```python
from build123d import *

# Parameters (mm, degrees)
SKETCH2_R           = 4.7625
BOSS_EXTRUDE1_DEPTH = 203.2
BOSS_EXTRUDE2_REACH = 30.575
SKETCH1_R           = 4.7625


with BuildPart() as part:
    # Sketch2 → Boss-Extrude1 (new body, symmetric)
    with BuildSketch(Plane(origin=(0, 0, 0), x_dir=(0, 0, -1), z_dir=(1, 0, 0))):
        with Locations((-23.8125, 0)):
            Circle(SKETCH2_R)
    extrude(amount=BOSS_EXTRUDE1_DEPTH, both=True)

    # Sketch1 → Boss-Extrude2 (add, up to next)
    with BuildSketch(Plane.XY, mode=Mode.PRIVATE) as boss_extrude2_sk1:
        with Locations((-155.575, 0)):
            Circle(SKETCH1_R)
    boss_extrude2_tool1 = extrude(boss_extrude2_sk1.sketch, amount=BOSS_EXTRUDE2_REACH, mode=Mode.PRIVATE) - part.part
    add(boss_extrude2_tool1.solids().sort_by_distance((-155.575, 0, 0))[0])
    # Sketch1 → Boss-Extrude2 (add, up to next)
    with BuildSketch(Plane.XY, mode=Mode.PRIVATE) as boss_extrude2_sk2:
        with Locations((155.575, 0)):
            Circle(SKETCH1_R)
    boss_extrude2_tool2 = extrude(boss_extrude2_sk2.sketch, amount=BOSS_EXTRUDE2_REACH, mode=Mode.PRIVATE) - part.part
    add(boss_extrude2_tool2.solids().sort_by_distance((155.575, 0, 0))[0])


solid = part.part
```
Work out the finished part from the listing and answer in its coordinate system (mm). A direction names the side the tool comes from. Coordinates: 2 decimals unless noted, no trailing zeros. Loops run counter-clockwise (first coordinate to the right, second up) from the corner with the lowest first, then second, coordinate; pieces in that order, holes last. Notation, with made-up numbers: (-18, 55) -> (-8, 55) arc R26 ccw to (-8, 84) -> close; hole circle Ø10 at (22.5, 65). An arc over 180 degrees is marked (long way). Answer as CSV lines item,"result".
Q1. A tool of negligible diameter and unlimited length cuts with its end or side. For faces 4 (the face through (2.84, 0.21, 28.57)), 5 (the face through (-160.333, 0.209, 9.094)), 6 (the face through (-156, 0, 0)), from which of +Z, -Z, +X, -X, +Y, -Y can it reach the whole face along a straight path? Write none if from no direction.
Findings:
face 4,"none"
face 5,"-Z"
face 6,"-Z, +X, -X, +Y, -Y"
Q2. The part is cut by section B-B on z = 9.5. Write down the section's boundary in (x, y) (1 decimal), and give its area (3 significant figures).
Findings:
outline,"circle Ø9.5 at (-155.6, 0); circle Ø9.5 at (155.6, 0)"
area,"143 mm²"
Q3. For a pull along X with two mould halves and no side action, classify faces 1 (the face through (203.2, 0, 24)), 2 (the face through (150.817, 0.209, 9.094)), 3 (the face through (156, 0, 0)) as +X half, -X half, draft (parallel to the pull), parting line (faces both ways), or undercut.
Findings:
face 1,"+X half"
face 2,"undercut"
face 3,"draft"
Q4. Each of these flat-tipped pins is pushed along its axis until it touches: pin 1 (2 mm diameter, centred on x = -117.5, z = 20.5, fed in from +Y); pin 2 (1 mm diameter, centred on y = 1, z = 10, fed in from -X); pin 3 (1 mm diameter, centred on x = -95.5, y = -2.5, fed in from +Z). Where does it stop, or does it pass through?
Findings:
pin 1,"stops at y = 4.16"
pin 2,"stops at x = -160.31"
pin 3,"stops at z = 28.13"
Q5. Find the intervals of material crossed by probe 1 along Z at (x, y) = (-82.5, 0.25); probe 2 along X at (y, z) = (2, 8.25); probe 3 along X at (y, z) = (1, 8.5), in increasing order.
Findings:
probe 1,"z = 19.06 to 28.57"
probe 2,"x = -159.9 to -151.25, 151.25 to 159.9"
probe 3,"x = -160.23 to -150.92, 150.92 to 160.23"
